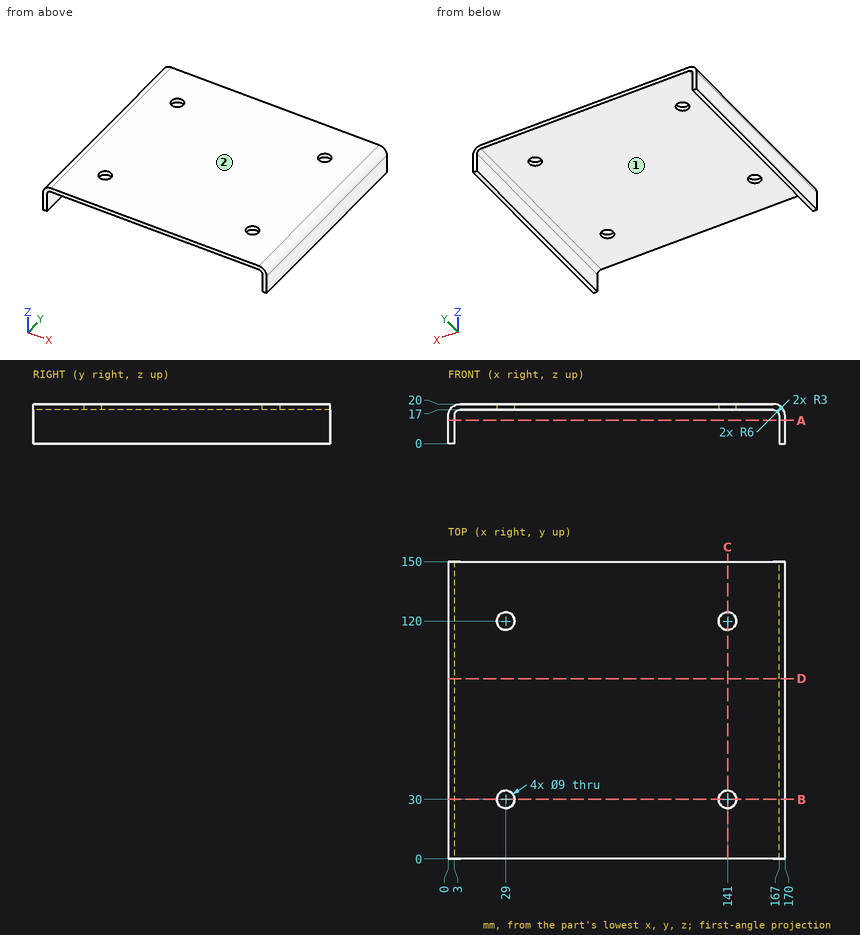
Drawing for the job (mm, zero at the part's lowest x, y, z). A direction names the side the tool comes from. Round coordinates to 2 decimals unless told otherwise and drop trailing zeros. Order: outer loops, then holes, each group sorted by start corner. A loop starts at its lowest first (then second) coordinate and runs counter-clockwise, first axis right, second up. Notation, with made-up numbers: M 68,37.25 L 111,37.25 A26 cw 111,53.25 Z; hole C 80,-14.5 d4. An arc over 180 degrees is marked long. Use one line per item in the form item = value.
Q1. Probe L1, parallel to Y at x = 29, z = 19.15; L2, parallel to X at y = 30, z = 19.2; L3, parallel to X at y = 90, z = 2. List the from-to ranges inside material, lowest first.
Recorded:
L1 = 0 to 25.5, 34.5 to 115.5, 124.5 to 150
L2 = 3.01 to 24.5, 33.5 to 136.5, 145.5 to 166.99
L3 = 0 to 3, 167 to 170
Q2. Saw through at C-C on x = 141. Give the cut face in (y, z), then the cut area to 3 significant figures.
Recorded:
outline = M 0,17 L 25.5,17 L 25.5,20 L 0,20 Z; M 34.5,17 L 115.5,17 L 115.5,20 L 34.5,20 Z; M 124.5,17 L 150,17 L 150,20 L 124.5,20 Z
area = 396 mm^2
Q3. Saw through at B-B on y = 30. Give the cut face in (x, z).
Recorded:
outline = M 0,0 L 3,0 L 3,14 A3 cw 6,17 L 24.5,17 L 24.5,20 L 6,20 A6 ccw 0,14 Z; M 33.5,17 L 136.5,17 L 136.5,20 L 33.5,20 Z; M 145.5,17 L 164,17 A3 cw 167,14 L 167,0 L 170,0 L 170,14 A6 ccw 164,20 L 145.5,20 Z
Q4. Saw through at A-A on z = 11.75. Give the cut face in (x, y).
Recorded:
outline = M 0,0 L 3,0 L 3,150 L 0,150 Z; M 167,0 L 170,0 L 170,150 L 167,150 Z
Q5. Which spindle directions (+Z, -Z, +X, -X, +Y, -Y) get a long thin tool onto all of the face, cutting with end or side? Do the marked faces 1 and 2. Say none if no direction does.
Recorded:
face_1 = -Z, +Y, -Y
face_2 = +Z, +X, -X, +Y, -Y
Q6. Saw through at D-D on y = 91. Give the cut face in (x, z).
Recorded:
outline = M 0,0 L 3,0 L 3,14 A3 cw 6,17 L 164,17 A3 cw 167,14 L 167,0 L 170,0 L 170,14 A6 ccw 164,20 L 6,20 A6 ccw 0,14 Z
Q7. Flat gauge pins, fed straight in: P1, Ø5.5, axis at x = 141, y = 120, coming from the -Z side; P2, Ø5, axis at y = 49.5, z = 17.5, coming from the -X side; P3, Ø1.5, axis at x = 87, y = 72, coming from the -Z side. Where does each tip first touch, or does it go through?
Recorded:
P1 = through
P2 = 0.08
P3 = 17
